from build123d import *

# Parameters (mm, degrees)
F0_R      = 1.25
F1_DEPTH  = 1.6
F2_W      = 3
F2_H      = 7
F2_W_2    = 6
F3_DEPTH  = 5
F4_DEPTH  = 8
F2_W_3    = 14
F2_H_2    = 16
F2_W_4    = 13
F5_DEPTH  = 29
F6_W      = 32
F6_H      = 29
F6_R      = 5
F6_R_2    = 4
F7_DEPTH  = 12
F9_DEPTH  = 32
F2_H_3    = 13
F2_W_5    = 17
F10_DEPTH = 26
F2_H_4    = 9
F11_DEPTH = 7
F2_W_6    = 19
F2_R      = 3.5
F2_R_2    = 4.5
F2_R_3    = 5
F2_R_4    = 3
F2_W_7    = 12
F12_DEPTH = 14
F2_W_8    = 15
F2_H_5    = 14
F13_DEPTH = 2
F2_H_6    = 22
F14_DEPTH = 25
F2_W_9    = 23
F2_H_7    = 23
F15_DEPTH = 23


with BuildPart() as f1:
    # F0 (on Top) → F1 (new body)
    with BuildSketch(Plane.XY):
        with BuildLine():
            Line((57.5, 42), (-61.5, 42))
            ThreePointArc((-61.5, 42), (-62.914214, 41.414214), (-63.5, 40))
            Line((-63.5, 40), (-63.5, -40))
            ThreePointArc((-63.5, -40), (-62.914214, -41.414214), (-61.5, -42))
            Line((-61.5, -42), (57.5, -42))
            ThreePointArc((57.5, -42), (58.914214, -41.414214), (59.5, -40))
            Line((59.5, -40), (59.5, 40))
            ThreePointArc((59.5, 40), (58.914214, 41.414214), (57.5, 42))
        make_face()
        with Locations((-40.5, -33)):
            Circle(F0_R, mode=Mode.SUBTRACT)
        with Locations((40.5, -33)):
            Circle(F0_R, mode=Mode.SUBTRACT)
        with Locations((-40.5, 33)):
            Circle(F0_R, mode=Mode.SUBTRACT)
        with Locations((40.5, 33)):
            Circle(F0_R, mode=Mode.SUBTRACT)
    extrude(amount=F1_DEPTH)

    # F2 (on face) → F3 (join)
    with BuildSketch(Plane.XY.offset(1.6)):
        with Locations((-65, 36.5)):
            Rectangle(F2_W, F2_H)
        with Locations((-60.5, 36.5)):
            Rectangle(F2_W_2, F2_H)
    extrude(amount=F3_DEPTH)

    # F2 (on face) → F4 (join)
    with BuildSketch(Plane.XY.offset(1.6)):
        with BuildLine():
            Line((-56.5, -17), (-63.5, -17))
            Line((-63.5, -17), (-63.5, -40))
            ThreePointArc((-63.5, -40), (-63.431852, -40.517638), (-63.232051, -41))
            Line((-63.232051, -41), (-56.5, -41))
            Line((-56.5, -41), (-56.5, -17))
        make_face()
        with BuildLine():
            Line((-63.5, -40), (-63.5, -17))
            Line((-63.5, -17), (-66.5, -17))
            Line((-66.5, -17), (-66.5, -41))
            Line((-66.5, -41), (-63.232051, -41))
            ThreePointArc((-63.232051, -41), (-63.431852, -40.517638), (-63.5, -40))
        make_face()
    extrude(amount=F4_DEPTH)

    # F2 (on face) → F5 (join)
    with BuildSketch(Plane.XY.offset(1.6)):
        with Locations((-70.5, 8)):
            Rectangle(F2_W_3, F2_H_2)
        with Locations((-57, 8)):
            Rectangle(F2_W_4, F2_H_2)
        with Locations((-70.5, -8)):
            Rectangle(F2_W_3, F2_H_2)
        with Locations((-57, -8)):
            Rectangle(F2_W_4, F2_H_2)
    extrude(amount=F5_DEPTH)

    # F6 (on face) → F7 (cut)
    with BuildSketch(Plane(origin=(-77.5, 0, 0), x_dir=(0, -1, 0), z_dir=(-1, 0, 0))):
        with Locations((0, 16.1)):
            Rectangle(F6_W, F6_H)
        with Locations((-8.5, 8.6)):
            Circle(F6_R, mode=Mode.SUBTRACT)
        with Locations((8.5, 8.6)):
            Circle(F6_R, mode=Mode.SUBTRACT)
        with Locations((-8.5, 23.6)):
            Circle(F6_R, mode=Mode.SUBTRACT)
        with Locations((8.5, 23.6)):
            Circle(F6_R, mode=Mode.SUBTRACT)
        with Locations((-8.5, 23.6)):
            Circle(F6_R_2)
        with Locations((8.5, 23.6)):
            Circle(F6_R_2)
        with Locations((-8.5, 8.6)):
            Circle(F6_R_2)
        with Locations((8.5, 8.6)):
            Circle(F6_R_2)
    extrude(amount=-F7_DEPTH, mode=Mode.SUBTRACT)

    # F8 (on face) → F9 (cut, through all)
    with BuildSketch(Plane(origin=(0, 16, 0), x_dir=(-1, 0, 0), z_dir=(0, 1, 0))):
        Polygon((50.5, 9.324275), (58, 30.6), (50.5, 30.6), align=None)
    extrude(amount=-F9_DEPTH, mode=Mode.SUBTRACT)

    # F2 (on face) → F10 (join)
    with BuildSketch(Plane.XY.offset(1.6)):
        with Locations((-65, 24.5)):
            Rectangle(F2_W, F2_H_3)
        with Locations((-55, 24.5)):
            Rectangle(F2_W_5, F2_H_3)
    extrude(amount=F10_DEPTH)

    # F2 (on face) → F11 (join)
    with BuildSketch(Plane.XY.offset(1.6)):
        with Locations((56.5, 33.5)):
            Rectangle(F2_W_2, F2_H_4)
        with Locations((61, 33.5)):
            Rectangle(F2_W, F2_H_4)
    extrude(amount=F11_DEPTH)

    # F2 (on face) → F12 (join)
    with BuildSketch(Plane.XY.offset(1.6)):
        with Locations((50, 19)):
            Rectangle(F2_W_6, F2_H_2)
        with Locations((61, 19)):
            Rectangle(F2_W, F2_H_2)
        with Locations((4.373364, 34.002684)):
            Circle(F2_R)
        with Locations((4.524074, 17)):
            Circle(F2_R_2)
        with Locations((18.344349, 13)):
            Rectangle(F2_W_4, F2_H_3)
        with Locations((33.176582, 10.356459)):
            Circle(F2_R_3)
        with Locations((15.981103, -1.763999)):
            Circle(F2_R_4)
        with Locations((1.36537, -1.763999)):
            Circle(F2_R_4)
        with Locations((7.36537, -34.65119)):
            Rectangle(F2_W_7, F2_H)
        with Locations((21.466679, -34.65119)):
            Rectangle(F2_W_7, F2_H)
    extrude(amount=F12_DEPTH)

    # F2 (on face) → F13 (join)
    with BuildSketch(Plane.XY.offset(1.6)):
        with Locations((52, 2)):
            Rectangle(F2_W_8, F2_H_5)
    extrude(amount=F13_DEPTH)

    # F2 (on face) → F14 (join)
    with BuildSketch(Plane.XY.offset(1.6)):
        with Locations((52, -25)):
            Rectangle(F2_W_8, F2_H_6)
        with Locations((61, -25)):
            Rectangle(F2_W, F2_H_6)
    extrude(amount=F14_DEPTH)

    # F2 (on face) → F15 (join)
    with BuildSketch(Plane.XY.offset(1.6)):
        with Locations((-21, 4.5)):
            Rectangle(F2_W_9, F2_H_7)
    extrude(amount=F15_DEPTH)


solid = f1.part
Input: part model. Units: mm. Frame: model coordinates. A direction names the side the tool comes from. Coordinates: 2 decimals unless noted, no trailing zeros. Loops run counter-clockwise (first coordinate to the right, second up) from the corner with the lowest first, then second, coordinate; pieces in that order, holes last.
(1) Material intervals for probe 1 along Y at (x, z) = (52.5, 2.5); probe 2 along Y at (x, z) = (40.5, 0.75); probe 3 along Z at (x, y) = (-75, 8.5), sorted ascending.
(2) Section D-D on x = -45. Return the cut outline in (y, z).
(3) Section C-C on y = -22.5. Return the cut outline in (x, z).
(4) Section B-B on x = -17.5. Return the cut outline in (y, z), then the cut area to 3 significant figures.
(5) Pull-direction query (X, two-part tool) for faces 1 (the face through (-71.584, -7.633, 19.695)), 2 (the face through (62.5, 19, 9)), 3 (the face through (13.365, -35, 9)); classes: released by +X, released by -X, zero draft, split by the parting line, or undercut.
(6) First-contact query: pin 1 Ø8 at (y, z) = (32, 8.5) entering from -X; pin 2 Ø17.5 at (x, y) = (56.5, 18.5) entering from +Z; pin 3 Ø2 at (x, y) = (-8, -13.5) entering from +Z. Flat tips, straight axial feed; report the tip coordinate or a pass-through.
(7) Set-up query: faces 4 (the face through (-46.5, 24, 14)), 5 (the face through (7, -35, 15.6)), 6 (the face through (-71.584, -11.188, 27.816)), 7 (the face through (3.94, 21.46, 8.5)). Return all of +Z, -Z, +X, -X, +Y, -Y with unobstructed straight access to the full face (end or side cutting, diameter ignored); none if empty.
(8) Section A-A on y = -8.5. Return the cut outline in (x, z), then the cut area to 3 significant figures.
Data:
1. probe 1: y = -36 to -14, -5 to 9, 11 to 27
1. probe 2: y = -42 to -34.25, -31.75 to 31.75, 34.25 to 42
1. probe 3: z = 3.6 to 4.6, 12.6 to 13.6, 18.6 to 19.6, 27.6 to 28.6
2. outline: (-42, 0) - (42, 0) - (42, 1.6) - (-42, 1.6) - close
3. outline: (-66.5, 1.6) - (-63.5, 1.6) - (-63.5, 0) - (59.5, 0) - (59.5, 1.6) - (62.5, 1.6) - (62.5, 26.6) - (44.5, 26.6) - (44.5, 1.6) - (-56.5, 1.6) - (-56.5, 9.6) - (-66.5, 9.6) - close
4. outline: (-42, 0) - (42, 0) - (42, 1.6) - (16, 1.6) - (16, 24.6) - (-7, 24.6) - (-7, 1.6) - (-42, 1.6) - close
4. area: 663 mm2
5. face 1: zero draft
5. face 2: released by +X
5. face 3: undercut
6. pin 1: stops at x = -66.5
6. pin 2: stops at z = 15.6
6. pin 3: stops at z = 1.6
7. face 4: +Z, +Y, -Y
7. face 5: +Z, -X, +Y, -Y
7. face 6: -X
7. face 7: +Z
8. outline: (-77.5, 3.6) - (-65.5, 3.6) - (-65.5, 1.6) - (-63.5, 1.6) - (-63.5, 0) - (59.5, 0) - (59.5, 1.6) - (-50.5, 1.6) - (-50.5, 9.32) - (-58, 30.6) - (-65.5, 30.6) - (-65.5, 28.6) - (-77.5, 28.6) - (-77.5, 27.6) - (-65.5, 27.6) - (-65.5, 19.6) - (-77.5, 19.6) - (-77.5, 18.6) - (-65.5, 18.6) - (-65.5, 13.6) - (-77.5, 13.6) - (-77.5, 12.6) - (-65.5, 12.6) - (-65.5, 4.6) - (-77.5, 4.6) - close
8. area: 600 mm2
